Autodesk Inventor part; units mm, degrees
ref_plane "YZ Plane" through (0, 0, 0) normal (1, 0, 0) x (0, 1, 0)
ref_plane "XZ Plane" through (0, 0, 0) normal (0, 1, 0) x (-1, 0, 0)
ref_plane "XY Plane" through (0, 0, 0) normal (0, 0, 1) x (1, 0, 0)
sketch "Sketch1" plane through (0, 0, 0) normal (0, 0, 1) x (1, 0, 0)
  circle A0 centre (0, 0) radius 5.7
  dimension "d0" = 11.4
extrude "Extrusion1" add sketch "Sketch1" along normal blind 20
chamfer "Chamfer1" distance 0.8 angle 45 1 edges at (-5.7, 0, 20)
sketch "Sketch2" plane through (0, 0, 0) normal (0, 0, 1) x (1, 0, 0)
  circle A0 centre (0, 0) radius 2.9
  dimension "d6" = 5.8
extrude "Extrusion2" cut sketch "Sketch2" along normal up to surface (20 mm away)
properties part number "Insert20mm"
Geometry check sheet. Reference: the model listing, model coordinates, mm. Round coordinates to 2 decimals unless told otherwise and drop trailing zeros. Loops run counter-clockwise (first coordinate to the right, second up) from the corner with the lowest first, then second, coordinate; pieces in that order, holes last.
Item 1: Cross-section at A-A on x = 0. Record the boundary of the cut face in (y, z).
Item 2: Mould release check, pull along Y, two halves, no side actions. Record for faces 1 (the cylindrical face through (-2.9, -0.1, 9.9)), 2 (the cylindrical face through (-4.5, 3.5, 9.5)), 3 (the flat face through (-0.1, -3.2, 20)): pulls with the +Y half, pulls with the -Y half, needs draft (parallel to the pull), parting line crosses it, or undercut.
Item 3: Thickness scan on line 1 (Y direction, x = 0, z = 4.5); line 2 (X direction, y = 1.5, z = 8.75). Record the ranges inside material, lowest first.
Item 4: Gauge pin test, flat end, axial feed: pin 1 (3 mm diameter, centred on x = -2, z = 16, fed in from +Y). Record the tip position at first contact, or that the pin passes through.
Item 5: Cross-section at C-C on z = 8.25. Record the boundary of the cut face in (x, y), then the cut area to 3 significant figures.
Answer sheet:
1. outline: (-5.7, 0) - (-2.9, 0) - (-2.9, 20) - (-4.9, 20) - (-5.7, 19.2) - close; (2.9, 0) - (5.7, 0) - (5.7, 19.2) - (4.9, 20) - (2.9, 20) - close
2. face 1: undercut
2. face 2: parting line crosses it
2. face 3: needs draft
3. line 1: y = -5.7 to -2.9, 2.9 to 5.7
3. line 2: x = -5.5 to -2.48, 2.48 to 5.5
4. pin 1: stops at y = 5.68
5. outline: circle Ø11.4 at (0, 0); hole circle Ø5.8 at (0, 0)
5. area: 75.6 mm2
